Here's how the part is built. I have some questions about the finished solid (model axes, mm). A direction names the side the tool comes from. Coordinates: 2 decimals unless noted, no trailing zeros. Write each loop counter-clockwise with the first axis right and the second up, starting at its lowest first coordinate (ties: lowest second). Pieces come first, ordered by that corner, then holes. Notation, with made-up numbers: (12.25, 40.25) -> (20.25, 40.25) arc R23 ccw to (20.25, 50.25) -> close; hole circle Ø11 at (-33.75, -36). An arc over 180 degrees is marked (long way). Answer in a Markdown table with one row per item. Add a question column.
from build123d import *

# Parameters (mm, degrees)
F1_DEPTH = 25.4
F3_DEPTH = 254
F4_W     = 25.4
F4_H     = 139.7
F4_H_2   = 25.4
F4_H_3   = 12.7
F4_W_2   = 63.5
F4_W_3   = 12.7
F4_H_4   = 254
F4_H_5   = 152.4
F4_H_6   = 101.6
F5_DEPTH = 203.2
F6_W     = 25.4
F6_H     = 76.2
F7_DEPTH = 101.6
F8_W     = 50.8
F8_H     = 152.4
F9_DEPTH = 25.4


with BuildPart() as f1:
    # F0 (on Top) → F1 (new body)
    with BuildSketch(Plane.XY):
        Polygon((-482.6, 0), (0, 0), (0, 279.4), (152.4, 279.4), (152.4, 482.6), (-482.6, 482.6), align=None)
    extrude(amount=F1_DEPTH)

    # F2 (on face) → F3 (join)
    with BuildSketch(Plane.XY.offset(25.4)):
        Polygon((152.4, 279.4), (152.4, 482.6), (-482.6, 482.6), (-482.6, 0), (0, 0), (0, 279.4), align=None)
        Polygon((-25.4, 25.4), (-457.2, 25.4), (-457.2, 457.2), (127, 457.2), (127, 304.8), (-25.4, 304.8), align=None, mode=Mode.SUBTRACT)
    extrude(amount=F3_DEPTH)

    # F4 (on face) → F5 (join)
    with BuildSketch(Plane.XY.offset(25.4)):
        with Locations((-190.5, 209.55)):
            Rectangle(F4_W, F4_H)
        with Locations((-368.3, 292.1)):
            Rectangle(F4_W, F4_H_2)
        with Locations((-190.5, 133.35)):
            Rectangle(F4_W, F4_H_3)
        with Locations((-234.95, 133.35)):
            Rectangle(F4_W_2, F4_H_3)
        with Locations((-146.05, 133.35)):
            Rectangle(F4_W_2, F4_H_3)
        with Locations((-273.05, 133.35)):
            Rectangle(F4_W_3, F4_H_3)
        with Locations((-107.95, 133.35)):
            Rectangle(F4_W_3, F4_H_3)
        with Locations((-368.3, 152.4)):
            Rectangle(F4_W, F4_H_4)
        Polygon((-355.6, 304.8), (-355.6, 279.4), (-203.2, 279.4), (-177.8, 279.4), (-25.4, 279.4), (-25.4, 304.8), align=None)
        with Locations((-368.3, 381)):
            Rectangle(F4_W, F4_H_5)
        with Locations((-107.95, 76.2)):
            Rectangle(F4_W_3, F4_H_6)
        with Locations((-273.05, 76.2)):
            Rectangle(F4_W_3, F4_H_6)
    extrude(amount=F5_DEPTH)

    # F6 (on face) → F7 (join)
    with BuildSketch(Plane.XY.offset(25.4)):
        with Locations((-9.9159989834, 342.9)):
            Rectangle(F6_W, F6_H)
    extrude(amount=F7_DEPTH)

    # F8 (on face) → F9 (cut)
    with BuildSketch(Plane.YZ.offset(-355.6)):
        with Locations((381, 101.6)):
            Rectangle(F8_W, F8_H)
    extrude(amount=-F9_DEPTH, mode=Mode.SUBTRACT)


solid = f1.part
Q1. I need wall thicknesses on line 1 (Y direction, x = -107.5, z = 199); line 2 (X direction, y = 271.5, z = 150); line 3 (Y direction, x = -305.5, z = 109). Which ranges of each line are inside material? Lowest first, please. Write a range as [from, to].
Q2. Imagine slicing it at A-A on y = 393. Please give me the cut outline in (x, z), plus the area to 3 significant figures.
Q3. For faces 1 (the flat face through (-368, 406.4, 101)), 2 (the flat face through (-111, 304.8, 151)), which set-ups out of +Z, -Z, +X, -X, +Y, -Y let a thin tool reach every point of the face, with its end or its side?
Q4. Imagine slicing it at B-B on z = 214. State how many separate pieces and enclosed holes the cut face has, plus the area to 3 significant figures.
Q5. If we mould it in two halves opening along X, with no side actions, what happens to faces 3 (the flat face through (-2, 260, 279.4)), 4 (the flat face through (152.4, 380, 138)), 5 (the flat face through (-355.6, 151, 126))? For each: pulls with the +X half, pulls with the -X half, needs draft (parallel to the pull), parting line crosses it, or undercut.
Q6. I'm going to push flat-ended pins straight in: P1, Ø12.5, axis at x = -5.5, y = 361, coming from the +Z side; P2, Ø10, axis at x = -265.5, y = 211.5, coming from the +Z side; P3, Ø8, axis at x = -372.5, y = 331, coming from the +Z side. Where does each tip first touch, or does it pass through?
Q7. Imagine slicing it at C-C on x = -423.5. Please give me the cut outline in (y, z).
Result sheet:
| question | item | result |
|---|---|---|
| 1 | line 1 | y = [0, 139.7], [279.4, 304.8], [457.2, 482.6] |
| 1 | line 2 | x = [-482.6, -457.2], [-381, -355.6], [-203.2, -177.8], [-25.4, 0] |
| 1 | line 3 | y = [0, 25.4], [279.4, 304.8], [457.2, 482.6] |
| 2 | outline | (-482.6, 0) -> (152.4, 0) -> (152.4, 279.4) -> (127, 279.4) -> (127, 25.4) -> (-457.2, 25.4) -> (-457.2, 279.4) -> (-482.6, 279.4) -> close; (-381, 177.8) -> (-355.6, 177.8) -> (-355.6, 228.6) -> (-381, 228.6) -> close |
| 2 | area | 30,300 mm^2 |
| 3 | face 1 | none |
| 3 | face 2 | +Z |
| 4 | separate pieces | 1 |
| 4 | enclosed holes | 5 |
| 4 | area | 81,900 mm^2 |
| 5 | face 3 | needs draft |
| 5 | face 4 | pulls with the +X half |
| 5 | face 5 | undercut |
| 6 | P1 | stops at z = 127 |
| 6 | P2 | stops at z = 25.4 |
| 6 | P3 | stops at z = 228.6 |
| 7 | outline | (0, 0) -> (482.6, 0) -> (482.6, 279.4) -> (457.2, 279.4) -> (457.2, 25.4) -> (25.4, 25.4) -> (25.4, 279.4) -> (0, 279.4) -> close |
